Here's how the part is built. I have some questions about the finished solid (model axes, mm). Coordinates: 2 decimals unless noted, no trailing zeros. Write each loop counter-clockwise with the first axis right and the second up, starting at its lowest first coordinate (ties: lowest second). Pieces come first, ordered by that corner, then holes. Notation, with made-up numbers: (16.5, -13) -> (37.5, -13) arc R14 cw to (37.5, 11) -> close; hole circle Ø10 at (16, -11). An arc over 180 degrees is marked (long way). Put each result on its own line as item: value. Start each with the question number.
Item 1: I want a section at B-B, the plane x = -114.3. List the corners of the cut face in (y, z) for me.
Item 2: I want a section at C-C, the plane z = 3.25. State how many separate pieces and enclosed holes the cut face has, then the cut area to 3 significant figures.
Item 3: I want a section at A-A, the plane x = 114.3. List the corners of the cut face in (y, z) for me, then the cut area to 3 significant figures.
Item 4: For pin 1 (17 mm diameter, centred on x = 190.5, y = -136.94, fed in from -Z), with a flat end and sliding along its axis, tell me the tip position at first contact or that it passes through.
Item 5: I want a section at D-D, the plane x = 33. List the corners of the cut face in (y, z) for me.
Item 6: I need wall thicknesses on line 1 (Y direction, x = 114.3, z = 4); line 2 (Y direction, x = -38.1, z = 4); line 3 (Y direction, x = 212.5, z = 3.75). Which ranges of each line are inside material? Lowest first, please. Write a range as [from, to].
from build123d import *

# Parameters (mm, degrees)
SKETCH1_W           = 533.4
SKETCH1_H           = 457.2
BOSS_EXTRUDE4_DEPTH = 6.35
SKETCH3_R           = 14.2875
CUT_EXTRUDE2_DEPTH  = 12.7


with BuildPart() as part:
    # Sketch1 → Boss-Extrude4 (new body)
    with BuildSketch(Plane.XY):
        Rectangle(SKETCH1_W, SKETCH1_H)
        with BuildLine():
            Line((-61.54804751, 145.902211593), (243.25195249, 145.902211593))
            ThreePointArc((243.25195249, 145.902211593), (255.95195249, 133.202211593), (243.25195249, 120.502211593))
            Line((243.25195249, 120.502211593), (-61.54804751, 120.502211593))
            ThreePointArc((-61.54804751, 120.502211593), (-74.24804751, 133.202211593), (-61.54804751, 145.902211593))
        make_face(mode=Mode.SUBTRACT)
        with BuildLine():
            Line((-61.54804751, 12.7), (243.25195249, 12.7))
            ThreePointArc((243.25195249, 12.7), (255.95195249, 0), (243.25195249, -12.7))
            Line((243.25195249, -12.7), (-61.54804751, -12.7))
            ThreePointArc((-61.54804751, -12.7), (-74.24804751, 0), (-61.54804751, 12.7))
        make_face(mode=Mode.SUBTRACT)
    extrude(amount=BOSS_EXTRUDE4_DEPTH)

    # Sketch3 → Cut-Extrude2 (cut)
    with BuildSketch(Plane(origin=(0, 0, 0), x_dir=(-1, 0, 0), z_dir=(0, 0, -1))):
        with Locations((-190.5, -136.944186205)):
            Circle(SKETCH3_R)
        with Locations((-114.3, -146.88837241)):
            Circle(SKETCH3_R)
        with Locations((-38.1, -156.832558615)):
            Circle(SKETCH3_R)
        with Locations((38.1, -166.77674482)):
            Circle(SKETCH3_R)
        with Locations((114.3, -176.720931025)):
            Circle(SKETCH3_R)
        with Locations((190.5, -186.66511723)):
            Circle(SKETCH3_R)
    extrude(amount=-CUT_EXTRUDE2_DEPTH, mode=Mode.SUBTRACT)


solid = part.part
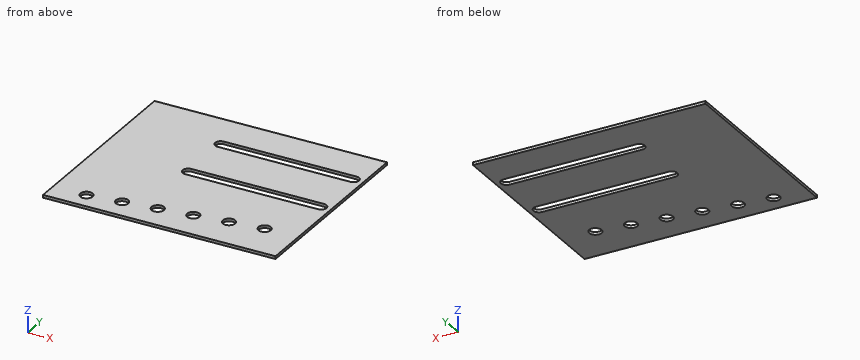
Calculated:
1. outline: (-228.6, 0) -> (-191.01, 0) -> (-191.01, 6.35) -> (-228.6, 6.35) -> close; (-162.43, 0) -> (228.6, 0) -> (228.6, 6.35) -> (-162.43, 6.35) -> close
2. separate pieces: 1
2. enclosed holes: 8
2. area: 224,000 mm2
3. outline: (-228.6, 0) -> (-161.18, 0) -> (-161.18, 6.35) -> (-228.6, 6.35) -> close; (-132.6, 0) -> (-12.7, 0) -> (-12.7, 6.35) -> (-132.6, 6.35) -> close; (12.7, 0) -> (120.5, 0) -> (120.5, 6.35) -> (12.7, 6.35) -> close; (145.9, 0) -> (228.6, 0) -> (228.6, 6.35) -> (145.9, 6.35) -> close
3. area: 2,400 mm2
4. pin 1: passes through
5. outline: (-228.6, 0) -> (-170.18, 0) -> (-170.18, 6.35) -> (-228.6, 6.35) -> close; (-143.49, 0) -> (-12.7, 0) -> (-12.7, 6.35) -> (-143.49, 6.35) -> close; (12.7, 0) -> (120.5, 0) -> (120.5, 6.35) -> (12.7, 6.35) -> close; (145.9, 0) -> (228.6, 0) -> (228.6, 6.35) -> (145.9, 6.35) -> close
6. line 1: y = [-228.6, -161.18], [-132.6, -12.7], [12.7, 120.5], [145.9, 228.6]
6. line 2: y = [-228.6, -181.06], [-152.49, -12.7], [12.7, 120.5], [145.9, 228.6]
6. line 3: y = [-228.6, -12.7], [12.7, 120.5], [145.9, 228.6]
